Check sheet for the modelled part. Datum: model origin and axes. Units: mm. A direction names the side the tool comes from. Coordinates: 2 decimals unless noted, no trailing zeros. Order: outer loops, then holes, each group sorted by start corner. A loop starts at its lowest first (then second) coordinate and runs counter-clockwise, first axis right, second up.
1. Draft check along X on faces 1 (the cylindrical face through (8.936, 3.759, 43.022)), 2 (the cylindrical face through (3.755, 12.325, 11.923)), 3 (the cylindrical face through (-8.936, 21.241, 43.629)). Enter one of: released by +X, released by -X, zero draft, split by the parting line, or undercut.
2. Cross-section at A-A (z = 0). Enter the section's corners in (x, y), then the cut area to 3 significant figures.
3. Thickness scan on line 1 (X direction, y = 17.75, z = 0); line 2 (Z direction, x = 5.5, y = 11.25); line 3 (X direction, y = 21.5, z = -8). Record the ranges inside material, lowest first.
4. Cross-section at B-B (x = 2). Enter the section's corners in (y, z), then the cut area to 3 significant figures.
5. Cross-section at C-C (y = 14.75). Enter the section's corners in (x, z).
6. Gauge pin test, flat ends, axial feed: pin 1 Ø3 at (y, z) = (17.5, 45.5) entering from -X; pin 2 Ø5 at (y, z) = (7, -14.5) entering from +X; pin 3 Ø2 at (x, y) = (-15.5, 20.5) entering from +Z. Record the tip position at first contact, or that the pin passes through.
7. Set-up check for faces 4 (the cylindrical face through (8.936, 21.241, 43.022)), 5 (the cylindrical face through (-8.936, 3.759, -43.022)), 6 (the cylindrical face through (-8.936, 21.241, -43.022)), 7 (the cylindrical face through (-8.936, 3.759, 43.629)): record each of +Z, -Z, +X, -X, +Y, -Y from which the full face is reachable in a straight line by a thin tool's end or side.
```python
from build123d import *

# Parameters (mm, degrees)
ESBO_O1_R                = 12.5
RESSALTO_EXTRUS_O1_DEPTH = 25
FILETE1_R                = 12.5


with BuildPart() as part:
    # Esboço1 → Ressalto-extrusão1 (new body)
    with BuildSketch(Plane(origin=(0, 0, 0), x_dir=(1, 0, 0), z_dir=(0, 1, 0))):
        with BuildLine():
            Line((-12.5, -21.650635095), (-12.5, -65))
            Line((-12.5, -65), (12.5, -65))
            Line((12.5, -65), (12.5, -21.650635095))
            ThreePointArc((12.5, -21.650635095), (25, 0), (12.5, 21.650635095))
            Line((12.5, 21.650635095), (12.5, 65))
            Line((12.5, 65), (-12.5, 65))
            Line((-12.5, 65), (-12.5, 21.650635095))
            ThreePointArc((-12.5, 21.650635095), (-25, 0), (-12.5, -21.650635095))
        make_face()
        with Locations(Location((0, 0, 0), (0, 0, 270))):
            Circle(ESBO_O1_R, mode=Mode.SUBTRACT)
    extrude(amount=RESSALTO_EXTRUS_O1_DEPTH)

    # Filete1
    filete1_edges = [part.edges().sort_by_distance(p)[0] for p in [
        (-12.5, 0, -43.325317547),
        (12.5, 0, -43.325317547),
        (-12.5, 25, -43.325317547),
        (12.5, 25, -43.325317547),
        (-12.5, 0, 43.325317547),
        (12.5, 0, 43.325317547),
        (12.5, 25, 43.325317547),
        (-12.5, 25, 43.325317547),
    ]]
    fillet(filete1_edges, radius=FILETE1_R - 0.0001)  # a hair under: the kernel refuses the full size


solid = part.part
```
Data:
1. face 1: released by +X
1. face 2: undercut
1. face 3: released by -X
2. outline: (-25, 0) - (-12.5, 0) - (-12.5, 25) - (-25, 25) - close; (12.5, 0) - (25, 0) - (25, 25) - (12.5, 25) - close
2. area: 625 mm2
3. line 1: x = -25 to -12.5, 12.5 to 25
3. line 2: z = -65 to -11.22, 11.22 to 65
3. line 3: x = -23.69 to -9.6, 9.6 to 23.69
4. outline: (0, -24.92) - (0.16, -24.92) - (0.16, -65) - (24.84, -65) - (24.84, -24.92) - (25, -24.92) - (25, -12.34) - (0, -12.34) - close; (0, 12.34) - (25, 12.34) - (25, 24.92) - (24.84, 24.92) - (24.84, 65) - (0.16, 65) - (0.16, 24.92) - (0, 24.92) - close
4. area: 2,610 mm2
5. outline: (-12.3, -65) - (12.3, -65) - (12.3, -21.77) arc R25 ccw to (12.3, 21.77) - (12.3, 65) - (-12.3, 65) - (-12.3, 21.77) arc R25 ccw to (-12.3, -21.77) - close; hole circle Ø25 at (0, 0)
6. pin 1: stops at x = -12
6. pin 2: stops at x = 21.93
6. pin 3: stops at z = 20.37
7. face 4: +Z, +X, +Y
7. face 5: -Z, -X, -Y
7. face 6: -Z, -X, +Y
7. face 7: +Z, -X, -Y
